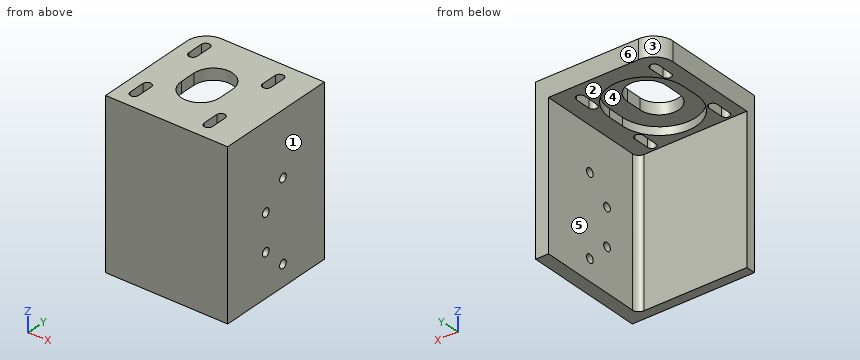
```python
from build123d import *

# Parameters (mm, degrees)
SKETCH1_W           = 38
SKETCH1_H           = 38
BOSS_EXTRUDE1_DEPTH = 6
BOSS_EXTRUDE2_DEPTH = 45
CUT_EXTRUDE1_DEPTH  = 6
CUT_EXTRUDE2_DEPTH  = 2.5
SKETCH6_R           = 1.3
CUT_EXTRUDE3_DEPTH  = 4
FILLET1_R           = 2
FILLET2_R           = 6


with BuildPart() as part:
    # Sketch1 → Boss-Extrude1 (new body)
    with BuildSketch(Plane.XY):
        with Locations((19, 19)):
            Rectangle(SKETCH1_W, SKETCH1_H)
    extrude(amount=BOSS_EXTRUDE1_DEPTH)

    # Sketch2 → Boss-Extrude2 (add)
    with BuildSketch(Plane(origin=(0, 0, 0), x_dir=(-1, 0, 0), z_dir=(0, 0, -1))):
        Polygon((-34, 38), (-34, 3), (0, 3), (0, 0), (-38, 0), (-38, 38), align=None)
    extrude(amount=BOSS_EXTRUDE2_DEPTH)

    # Sketch3 → Cut-Extrude1 (cut)
    with BuildSketch(Plane.XY.offset(6)):
        with BuildLine():
            Line((6.3, 33), (6.3, 28))
            ThreePointArc((6.3, 28), (5, 26.7), (3.7, 28))
            Line((3.7, 28), (3.7, 33))
            ThreePointArc((3.7, 33), (5, 34.3), (6.3, 33))
        make_face()
        with BuildLine():
            Line((29.3, 33), (29.3, 28))
            ThreePointArc((29.3, 28), (28, 26.7), (26.7, 28))
            Line((26.7, 28), (26.7, 33))
            ThreePointArc((26.7, 33), (28, 34.3), (29.3, 33))
        make_face()
        with BuildLine():
            Line((6.3, 10), (6.3, 5))
            ThreePointArc((6.3, 5), (5, 3.7), (3.7, 5))
            Line((3.7, 5), (3.7, 10))
            ThreePointArc((3.7, 10), (5, 11.3), (6.3, 10))
        make_face()
        with BuildLine():
            Line((29.3, 10), (29.3, 5))
            ThreePointArc((29.3, 5), (28, 3.7), (26.7, 5))
            Line((26.7, 5), (26.7, 10))
            ThreePointArc((26.7, 10), (28, 11.3), (29.3, 10))
        make_face()
        with BuildLine():
            Line((22.5, 21.5), (22.5, 16.5))
            ThreePointArc((22.5, 16.5), (16.5, 10.5), (10.5, 16.5))
            Line((10.5, 16.5), (10.5, 21.5))
            ThreePointArc((10.5, 21.5), (16.5, 27.5), (22.5, 21.5))
        make_face()
    extrude(amount=-CUT_EXTRUDE1_DEPTH, mode=Mode.SUBTRACT)

    # Sketch5 → Cut-Extrude2 (cut)
    with BuildSketch(Plane(origin=(0, 0, 0), x_dir=(-1, 0, 0), z_dir=(0, 0, -1))):
        with BuildLine():
            Line((-5, 21.5), (-5, 16.5))
            ThreePointArc((-5, 16.5), (-16.5, 5), (-28, 16.5))
            Line((-28, 16.5), (-28, 21.5))
            ThreePointArc((-28, 21.5), (-16.5, 33), (-5, 21.5))
        make_face()
    extrude(amount=-CUT_EXTRUDE2_DEPTH, mode=Mode.SUBTRACT)

    # Sketch6 → Cut-Extrude3 (cut)
    with BuildSketch(Plane(origin=(38, 0, 0), x_dir=(0, 0, -1), z_dir=(1, 0, 0))):
        with Locations((13.582485579, 21.717514421)):
            Circle(SKETCH6_R)
        with Locations((20.3, 15)):
            Circle(SKETCH6_R)
        with Locations((38.417514421, 21.717514421)):
            Circle(SKETCH6_R)
        with Locations((31.7, 15)):
            Circle(SKETCH6_R)
    extrude(amount=-CUT_EXTRUDE3_DEPTH, mode=Mode.SUBTRACT)

    # Fillet1
    fillet1_edges = [part.edges().sort_by_distance(p)[0] for p in [
        (34, 3, -22.5),
    ]]
    fillet(fillet1_edges, radius=FILLET1_R)

    # Fillet2
    fillet2_edges = [part.edges().sort_by_distance(p)[0] for p in [
        (0, 38, 3),
    ]]
    fillet(fillet2_edges, radius=FILLET2_R)


solid = part.part
```
For this review, take the finished solid that the model builds, in its own axes (mm). Face numbers are marked on the shaded views. A direction names the side the tool comes from. Round coordinates to 2 decimals unless told otherwise and drop trailing zeros. Write each loop counter-clockwise with the first axis right and the second up, starting at its lowest first coordinate (ties: lowest second). Pieces come first, ordered by that corner, then holes. Notation, with made-up numbers: (43, 23) - (71, 23) arc R18 ccw to (71, 29) - close; hole circle Ø9 at (7, 39.5). An arc over 180 degrees is marked (long way). Write each question's results on one line, items separated by ' | '.
Item 1: For the marked faces 5 and 6, list the 3-axis set-ups (+Z, -Z, +X, -X, +Y, -Y) from which the entire face can be reached by the end or side of a thin tool; tool diameter is ignored.
Calculated:
face 5: -Z, -X, +Y | face 6: +Z, -Z, +X, -X, +Y
Item 2: To check wall thickness, follow line 1 along X through (y, z) = (6, 3); line 2 along Y through (x, z) = (22.5, -8); line 3 along X through (y, z) = (21, -11). State the ranges of each line that lie inside material, in increasing order. Write a range as from..to.
Calculated:
line 1: x = 0..3.7, 6.3..26.7, 29.3..38 | line 2: y = 0..3 | line 3: x = 34..38
Item 3: Take a section at A-A on x = 16.5. State the section outline as (y, z) points, then the cut area to 4 significant figures.
Calculated:
outline: (0, -45) - (3, -45) - (3, 0) - (5, 0) - (5, 2.5) - (10.5, 2.5) - (10.5, 6) - (0, 6) - close; (27.5, 2.5) - (33, 2.5) - (33, 0) - (38, 0) - (38, 6) - (27.5, 6) - close | area: 233.5 mm^2
Item 4: For pin 1 (3 mm diameter, centred on y = 26, z = -15, fed in from -X); pin 2 (4 mm diameter, centred on x = 8.5, y = 8, fed in from -Z), all flat-tipped, find the tip position at first contact; note any pin that passes through.
Calculated:
pin 1: stops at x = 34 | pin 2: stops at z = 0
Item 5: Draft analysis for pull direction X (two halves, no side actions). For the marked faces 1, 2, 3 and 4, state which applies: pulls with the +X half, pulls with the -X half, needs draft (parallel to the pull), parting line crosses it, or undercut.
Calculated:
face 1: pulls with the +X half | face 2: needs draft | face 3: pulls with the -X half | face 4: undercut
Item 6: Take a section at C-C on y = 7. State the section outline as (x, z) points, then the cut area to 3 significant figures.
Calculated:
outline: (0, 0) - (3.7, 0) - (3.7, 6) - (0, 6) - close; (6.3, 0) - (10.02, 0) - (10.02, 2.5) - (22.98, 2.5) - (22.98, 0) - (26.7, 0) - (26.7, 6) - (6.3, 6) - close; (29.3, 0) - (34, 0) - (34, -45) - (38, -45) - (38, 6) - (29.3, 6) - close | area: 344 mm^2
Item 7: Take a section at B-B on z = -31.7. State the section outline as (x, y) points.
Calculated:
outline: (0, 0) - (38, 0) - (38, 13.7) - (34, 13.7) - (34, 5) arc R2 cw to (32, 3) - (0, 3) - close; (34, 16.3) - (38, 16.3) - (38, 38) - (34, 38) - close
Item 8: Take a section at D-D on z = -24.5. State the section outline as (x, y) points.
Calculated:
outline: (0, 0) - (38, 0) - (38, 38) - (34, 38) - (34, 5) arc R2 cw to (32, 3) - (0, 3) - close
